```python
from build123d import *

# Parameters (mm, degrees)
AUFSATZ_LINEAR_AUSTRAGEN1_DEPTH = 1.3
VERRUNDUNG1_R                   = 0.5
KREISMUSTER1_COUNT              = 10
VERRUNDUNG1_OF_KREISMUSTER1_R   = 0.5
FASE1_SIZE2                     = 0.2
FASE1_SIZE                      = 0.274584275
FASE1_EDGE_2_SIZE               = 0.2
FASE1_EDGE_3_SIZE               = 0.2
FASE1_EDGE_4_SIZE               = 0.2
FASE1_EDGE_5_SIZE               = 0.2


with BuildPart() as part:
    # Skizze1 → Rotation1 (revolve)
    with BuildSketch(Plane(origin=(0, 0, 0), x_dir=(0, 0, -1), z_dir=(1, 0, 0))):
        Polygon((0, 2), (-4.66, 2), (-4.66, 3.001343994), (-2.66, 3.5), (-1.66, 3.5), (-1.66, 6), (0, 6), (1.3, 6), (1.3, 4.57), (0, 4.57), align=None)
    revolve(axis=Axis((0, 0, 23.408695652), (0, 0, -1)))

    # Skizze4 → Aufsatz-Linear austragen1 (add)
    with BuildSketch(Plane(origin=(0, 0, 0), x_dir=(-1, 0, 0), z_dir=(0, 0, -1))):
        with BuildLine():
            Line((-0.808470756, 3.57), (-1.2, 4.409637173))
            ThreePointArc((-1.2, 4.409637173), (0, 4.57), (1.2, 4.409637173))
            Line((1.2, 4.409637173), (0.808470756, 3.57))
            Line((0.808470756, 3.57), (-0.808470756, 3.57))
        make_face()
    aufsatz_linear_austragen1 = extrude(amount=AUFSATZ_LINEAR_AUSTRAGEN1_DEPTH)

    # Verrundung1
    verrundung1_edges = [part.edges().sort_by_distance(p)[0] for p in [
        (-0.808470756, 3.57, -0.65),
        (0.808470756, 3.57, -0.65),
    ]]
    fillet(verrundung1_edges, radius=VERRUNDUNG1_R)

    # Kreismuster1: Aufsatz-Linear austragen1 ×10 about axis
    kreismuster1_axis = Axis((0, 0, 0), (0, 0, 1))
    for i in range(1, KREISMUSTER1_COUNT):
        add(aufsatz_linear_austragen1.rotate(kreismuster1_axis, i * 360 / KREISMUSTER1_COUNT))

    # Verrundung1 of Kreismuster1
    verrundung1_of_kreismuster1_edges = [part.edges().sort_by_distance(p)[0] for p in [
        (-2.752459932, 2.412983483, -0.65),
        (-1.44432677, 3.363397857, -0.65),
        (-3.645102966, 0.334289289, -0.65),
        (-3.14544056, 1.872092051, -0.65),
        (-3.14544056, -1.872092051, -0.65),
        (-3.645102966, -0.334289289, -0.65),
        (-1.44432677, -3.363397857, -0.65),
        (-2.752459932, -2.412983483, -0.65),
        (0.808470756, -3.57, -0.65),
        (-0.808470756, -3.57, -0.65),
        (2.752459932, -2.412983483, -0.65),
        (1.44432677, -3.363397857, -0.65),
        (3.645102966, -0.334289289, -0.65),
        (3.14544056, -1.872092051, -0.65),
        (3.14544056, 1.872092051, -0.65),
        (3.645102966, 0.334289289, -0.65),
        (1.44432677, 3.363397857, -0.65),
        (2.752459932, 2.412983483, -0.65),
    ]]
    fillet(verrundung1_of_kreismuster1_edges, radius=VERRUNDUNG1_OF_KREISMUSTER1_R)

    # Skizze5 → Schnitt-Rotation1 (revolve, cut)
    with BuildSketch(Plane(origin=(0, 0, 0), x_dir=(0, 0, -1), z_dir=(1, 0, 0))):
        with BuildLine():
            Line((0.5, 6), (0.5, 5))
            Line((0.5, 5), (1.153553391, 4.346446609))
            ThreePointArc((1.153553391, 4.346446609), (1.261939766, 4.184234935), (1.3, 3.992893219))
            Line((1.3, 3.992893219), (1.3, 2.59724793))
            Line((1.3, 2.59724793), (2.535311957, 2.59724793))
            Line((2.535311957, 2.59724793), (2.535311957, 6))
            Line((2.535311957, 6), (0.5, 6))
        make_face()
    revolve(axis=Axis((0, 0, -4.981936438), (0, 0, 1)), mode=Mode.SUBTRACT)

    # Fase1
    fase1_edges = [part.edges().sort_by_distance(p)[0] for p in [
        (0, -3.001343994, 4.66),
    ]]
    chamfer(fase1_edges, length=FASE1_SIZE, length2=FASE1_SIZE2)

    # Fase1 edge 2
    fase1_edge_2_edges = [part.edges().sort_by_distance(p)[0] for p in [
        (0, -2, 4.66),
    ]]
    chamfer(fase1_edge_2_edges, length=FASE1_EDGE_2_SIZE)

    # Fase1 edge 3
    fase1_edge_3_edges = [part.edges().sort_by_distance(p)[0] for p in [
        (0, -2, 0),
    ]]
    chamfer(fase1_edge_3_edges, length=FASE1_EDGE_3_SIZE)

    # Fase1 edge 4
    fase1_edge_4_edges = [part.edges().sort_by_distance(p)[0] for p in [
        (0, -6, -0.5),
    ]]
    chamfer(fase1_edge_4_edges, length=FASE1_EDGE_4_SIZE)

    # Fase1 edge 5
    fase1_edge_5_edges = [part.edges().sort_by_distance(p)[0] for p in [
        (0, -6, 1.66),
    ]]
    chamfer(fase1_edge_5_edges, length=FASE1_EDGE_5_SIZE)


solid = part.part
```
Verification items for the finished model (mm, model axes). A direction names the side the tool comes from. Round coordinates to 2 decimals unless told otherwise and drop trailing zeros. Write each loop counter-clockwise with the first axis right and the second up, starting at its lowest first coordinate (ties: lowest second). Pieces come first, ordered by that corner, then holes. Notation, with made-up numbers: (-31.5, -30) - (0.5, -30) arc R20 cw to (0.5, -26) - close; hole circle Ø1 at (48.25, 26.5). An arc over 180 degrees is marked (long way). Answer as a JSON object with one key per item and string values. Group by question number.
Q1. Tool access check on faces 5 (the flat face through (3.397, -1.097, -0.641)), 6 (the flat face through (-2.28, -3.09, -1.3)). Record the directions out of +Z, -Z, +X, -X, +Y, -Y that give a thin tool (end or side, any length) a straight path to the whole face; none if there is none.
Q2. Go/stop test with flat-tipped pins: pin 1 Ø2 at (y, z) = (-1.5, 0.5) entering from -X; pin 2 Ø2 at (x, z) = (2.5, 2) entering from -Y; pin 3 Ø2 at (y, z) = (5, 1) entering from +X; pin 4 Ø2.5 at (x, y) = (0, 0) entering from -Z. Record where each tip stops, or that it passes through.
Q3. Thickness scan on line 1 (X direction, y = 4, z = -0.15); line 2 (X direction, y = 0, z = 2.2); line 3 (Y direction, x = -2.75, z = 4). Record the ranges inside material, lowest first.
Q4. Mould release check, pull along X, two halves, no side actions. Record for faces 1 (the flat face through (-3.397, 1.097, -0.641)), 2 (the flat face through (-5, 2, -0.5)), 3 (the cylindrical face through (-1.341, 3.233, 2.153)), 4 (the flat face through (0, 3.57, -1)): released by +X, released by -X, zero draft, split by the parting line, or undercut.
Q5. Section check C-C, the plane z = 3.25. Enter the section's corners in (x, y), plus the area to 3 significant figures.
Found:
{
 "1": {"face 5": "-Z", "face 6": "-Z, +X, -X, +Y, -Y"},
 "2": {"pin 1": "stops at x = -5.98", "pin 2": "stops at y = -5.77", "pin 3": "stops at x = 4.47", "pin 4": "passes through"},
 "3": {"line 1": "x = -4.47 to -1.57, -1.01 to 1.01, 1.57 to 4.47", "line 2": "x = -3.5 to -2, 2 to 3.5", "line 3": "y = -1.57 to 1.57"},
 "4": {"face 1": "undercut", "face 2": "zero draft", "face 3": "split by the parting line", "face 4": "undercut"},
 "5": {"outline": "circle Ø6.71 at (0, 0); hole circle Ø4 at (0, 0)", "area": "22.8 mm^2"}
}
